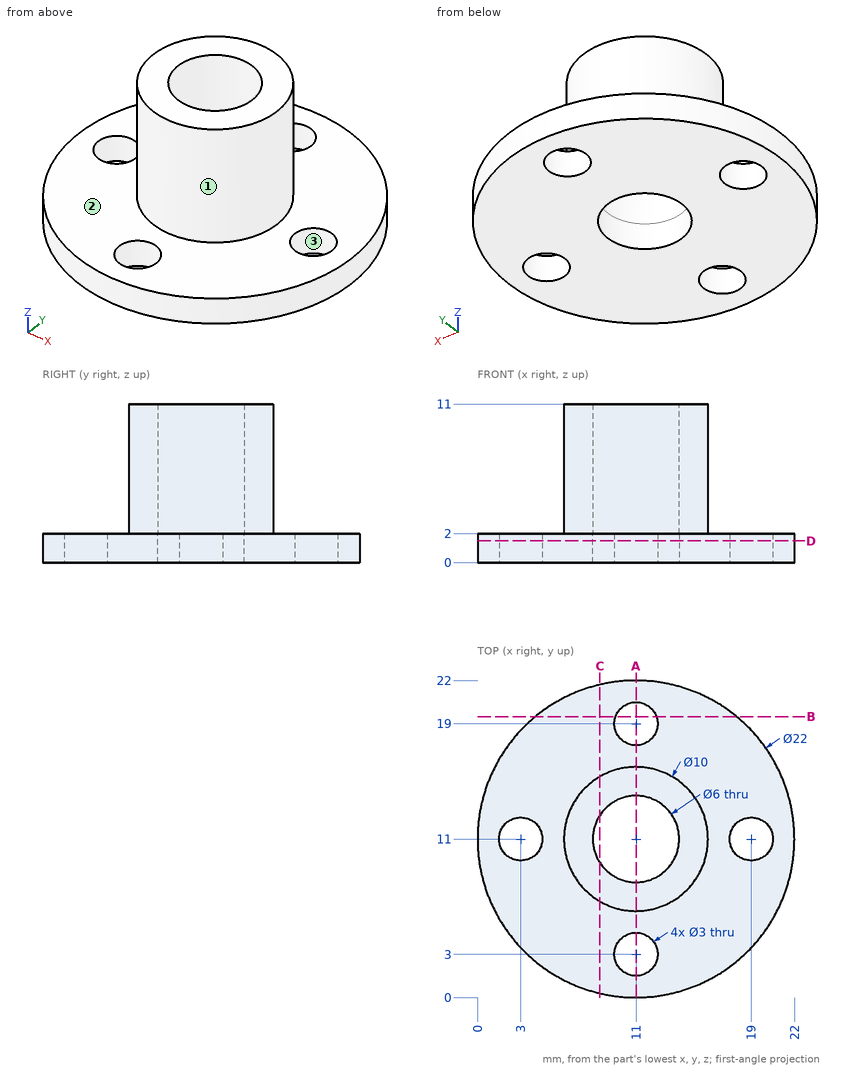
The figure shows three views and two pictorial views of one solid part (mm, origin at its lowest corner). Answer the questions. Give positions to 0.01 mm unless a question says otherwise; leave off trailing zeros. Order: outer loops, then holes, each group sorted by start corner. A loop starts at its lowest first (then second) coordinate and runs counter-clockwise, first axis right, second up. Notation, with made-up numbers: M 71.5,9 L 106.5,9 A21 ccw 106.5,22 Z; hole C 85,16.25 d9. An arc over 180 degrees is marked long. Return JSON: item names as keys, results as strings.
Q1. Find the intervals of material crossed by line 1 along Y through (x, z) = (11, 0.45); line 2 along Z through (x, y) = (19.5, 5); line 3 along X through (y, z) = (8.25, 3.75), in increasing order. Write a range as [from, to].
Answer below:
{"line 1": "y = [0, 1.5], [4.5, 8], [14, 17.5], [20.5, 22]", "line 2": "z = [0, 2]", "line 3": "x = [6.82, 9.8], [12.2, 15.18]"}
Q2. Find section C-C, the plane x = 8.5. Write down the section's boundary in (y, z), and give its area (3 significant figures).
Answer below:
{"outline": "M 0.29,0 L 9.34,0 L 9.34,11 L 6.67,11 L 6.67,2 L 0.29,2 Z; M 12.66,0 L 21.71,0 L 21.71,2 L 15.33,2 L 15.33,11 L 12.66,11 Z", "area": "84.3 mm^2"}
Q3. Find section B-B, the plane y = 19.5. Write down the section's boundary in (x, z), and give its area (3 significant figures).
Answer below:
{"outline": "M 4.02,0 L 9.59,0 L 9.59,2 L 4.02,2 Z; M 12.41,0 L 17.98,0 L 17.98,2 L 12.41,2 Z", "area": "22.3 mm^2"}
Q4. Find section A-A, the plane x = 11. Write down the section's boundary in (y, z).
Answer below:
{"outline": "M 0,0 L 1.5,0 L 1.5,2 L 0,2 Z; M 4.5,0 L 8,0 L 8,11 L 6,11 L 6,2 L 4.5,2 Z; M 14,0 L 17.5,0 L 17.5,2 L 16,2 L 16,11 L 14,11 Z; M 20.5,0 L 22,0 L 22,2 L 20.5,2 Z"}
Q5. Find section D-D, the plane z = 1.5. Write down the section's boundary in (x, y).
Answer below:
{"outline": "C 11,11 d22; hole C 3,11 d3; hole C 11,11 d6; hole C 11,3 d3; hole C 11,19 d3; hole C 19,11 d3"}
Q6. The mould has two halves that part along X. Classify the marked faces 1, 2 and 3: pulls with the +X half, pulls with the -X half, needs draft (parallel to the pull), parting line crosses it, or undercut.
Answer below:
{"face 1": "parting line crosses it", "face 2": "needs draft", "face 3": "undercut"}
Q7. Each of these flat-tipped pins is pushed along its axis until it touches: pin 1 (3.5 mm diameter, centred on x = 11, y = 19, fed in from +Z); pin 2 (1.5 mm diameter, centred on x = 3.5, z = 1.5, fed in from +Y); pin 3 (1.5 mm diameter, centred on x = 15, z = 3, fed in from +Y). Where does it stop, or does it pass through?
Answer below:
{"pin 1": "stops at z = 2", "pin 2": "stops at y = 19.69", "pin 3": "stops at y = 14.8"}
